Can you work these out from the model? Positions are in its coordinate system, mm. A direction names the side the tool comes from. Coordinates: 2 decimals unless noted, no trailing zeros. Order: outer loops, then holes, each group sorted by start corner. A loop starts at its lowest first (then second) coordinate and runs counter-clockwise, first axis right, second up. Notation, with made-up numbers: (-29.75, 76.25) -> (10.25, 76.25) arc R30 ccw to (10.25, 111.25) -> close; hole circle Ø9 at (18, 2.5). An arc over 180 degrees is marked (long way). Answer in a Markdown table with one row per item. Add a question column.
1. Will these pins go through, and if not, where does the flat tip stop? pin 1 (2 mm diameter, centred on x = 0, z = -1.5, fed in from -Y); pin 2 (1 mm diameter, centred on x = -0.5, z = 0.5, fed in from +Y).
2. On a 3-axis mill with a long thin cutter (end or side, diameter ignored), from which of +Z, -Z, +X, -X, +Y, -Y can I reach the whole of each face in a straight line? I mean faces 1 (the face through (-0.59, 7.61, -4.46)), 2 (the face through (0, 0.8, 0)). Say none if no direction works.
3. If I drill on line 1 along Z through (x, y) = (0, 7.7); line 2 along Y through (x, z) = (1.5, 1), over which ranges is the centre line in solid material (lowest first)? Write a range as [from, to].
4. We'd pull the mould along X, two halves only. Please class faces 3 (the face through (-1.08, 3.94, 4.88)), 4 (the face through (-0.59, 0.39, 4.46)): pulls with the +X half, pulls with the -X half, needs draft (parallel to the pull), parting line crosses it, or undercut.
5. Imagine slicing it at A-A on x = 0. Write out the boundary of the cut face in (y, z).
6. Imagine slicing it at C-C on y = 4.75. Write out the boundary of the cut face in (x, z).
7. Imagine slicing it at B-B on z = 0. Write out the boundary of the cut face in (x, y).
from build123d import *

# Parameters (mm, degrees)
SCHIZZO1_R                   = 5
ESTRUSIONE_ESTRUSIONE1_DEPTH = 8
SCHIZZO2_R                   = 4.5
TAGLIO_ESTRUSIONE1_DEPTH     = 0.8
SCHIZZO3_R                   = 4.5
TAGLIO_ESTRUSIONE2_DEPTH     = 0.8


with BuildPart() as part:
    # Schizzo1 → Estrusione-Estrusione1 (new body)
    with BuildSketch(Plane(origin=(0, 0, 0), x_dir=(1, 0, 0), z_dir=(0, 1, 0))):
        Circle(SCHIZZO1_R)
    extrude(amount=ESTRUSIONE_ESTRUSIONE1_DEPTH)

    # Schizzo2 → Taglio-Estrusione1 (cut)
    with BuildSketch(Plane(origin=(0, 8, 0), x_dir=(1, 0, 0), z_dir=(0, 1, 0))):
        Circle(SCHIZZO2_R)
    extrude(amount=-TAGLIO_ESTRUSIONE1_DEPTH, mode=Mode.SUBTRACT)

    # Schizzo3 → Taglio-Estrusione2 (cut)
    with BuildSketch(Plane.XZ):
        Circle(SCHIZZO3_R)
    extrude(amount=-TAGLIO_ESTRUSIONE2_DEPTH, mode=Mode.SUBTRACT)


solid = part.part
Answers follow:
| question | item | result |
|---|---|---|
| 1 | pin 1 | stops at y = 0.8 |
| 1 | pin 2 | stops at y = 7.2 |
| 2 | face 1 | +Y |
| 2 | face 2 | -Y |
| 3 | line 1 | z = [-5, -4.5], [4.5, 5] |
| 3 | line 2 | y = [0.8, 7.2] |
| 4 | face 3 | parting line crosses it |
| 4 | face 4 | undercut |
| 5 | outline | (0, -5) -> (8, -5) -> (8, -4.5) -> (7.2, -4.5) -> (7.2, 4.5) -> (8, 4.5) -> (8, 5) -> (0, 5) -> (0, 4.5) -> (0.8, 4.5) -> (0.8, -4.5) -> (0, -4.5) -> close |
| 6 | outline | circle Ø10 at (0, 0) |
| 7 | outline | (-5, 0) -> (-4.5, 0) -> (-4.5, 0.8) -> (4.5, 0.8) -> (4.5, 0) -> (5, 0) -> (5, 8) -> (4.5, 8) -> (4.5, 7.2) -> (-4.5, 7.2) -> (-4.5, 8) -> (-5, 8) -> close |
